Autodesk Inventor part; units mm, degrees
ref_plane "YZ Plane" through (0, 0, 0) normal (1, 0, 0) x (0, 1, 0)
ref_plane "XZ Plane" through (0, 0, 0) normal (0, 1, 0) x (-1, 0, 0)
ref_plane "XY Plane" through (0, 0, 0) normal (0, 0, 1) x (1, 0, 0)
sketch "本体面" plane through (0, 0, 0) normal (0, 0, 1) x (1, 0, 0)
  line L0 (-13.7, 10) -> (13.7, 10)
  line L1 (13.7, 10) -> (13.7, 0)
  line L2 (13.7, 0) -> (-13.7, 0)
  line L3 (-13.7, 0) -> (-13.7, 10)
  point P0 (0, 0)
  point P1 (0, 0)
  dimension "d0" = 27.4
  dimension "d1" = 10
extrude "本体" add sketch "本体面" along normal blind 42
sketch "空洞面" plane through (0, 0, 42) normal (0, 0, 1) x (1, 0, 0)
  line L0 (-11.9, 10) -> (11.9, 10)
  line L1 (11.9, 10) -> (11.9, 3.5)
  line L2 (9.9, 1.5) -> (-9.9, 1.5)
  line L3 (-11.9, 3.5) -> (-11.9, 10)
  line L4 (13.7, 10) -> (-13.7, 10)
  arc A0 (-11.9, 3.5) -> (-9.9, 1.5) centre (-9.9, 3.5) ccw
  arc A1 (9.9, 1.5) -> (11.9, 3.5) centre (9.9, 3.5) ccw
  point P0 (0, 0)
  point P1 (11.9, 1.5)
  point P2 (-11.9, 1.5)
  point P3 (0, 10)
  dimension "d4" = 23.8
  dimension "d5" = 8.5
  dimension "d6" = 2
extrude "空洞" cut sketch "空洞面" against normal blind 42
sketch "左溝面" plane through (0, 0, 42) normal (0, 0, 1) x (1, 0, 0)
  line L0 (-12.9, 9.2) -> (-11.9, 9.2)
  line L1 (-11.9, 9.2) -> (-11.9, 7.2)
  line L2 (-11.9, 7.2) -> (-12.9, 7.2)
  line L3 (-12.9, 7.2) -> (-12.9, 9.2)
  line L4 (-11.9, 10) -> (-13.7, 10) construction
  line L5 (-13.7, 10) -> (-13.7, 0) construction
  line L6 (-11.9, 3.5) -> (-11.9, 10) construction
  point P0 (0, 0)
  dimension "d10" = 2
  dimension "d27" = 0.8
  dimension "d28" = 0.8
extrude "左溝" cut sketch "左溝面" against normal blind 41
sketch "右溝面" plane through (0, 0, 42) normal (0, 0, 1) x (1, 0, 0)
  line L0 (11.9, 9.2) -> (12.9, 9.2)
  line L1 (12.9, 9.2) -> (12.9, 7.2)
  line L2 (12.9, 7.2) -> (11.9, 7.2)
  line L3 (11.9, 7.2) -> (11.9, 9.2)
  line L4 (13.7, 10) -> (11.9, 10)
  line L5 (13.7, 0) -> (13.7, 10)
  line L6 (11.9, 10) -> (11.9, 3.5)
  point P0 (0, 0)
  dimension "d22" = 2
  dimension "d29" = 0.8
  dimension "d30" = 0.8
extrude "右溝" cut sketch "右溝面" against normal blind 41
sketch "右穴位置" plane through (13.7, 0, 0) normal (1, 0, 0) x (0, 0, -1)
  line L0 (-20, 0) -> (0, 0) construction
  line L1 (-20, 0) -> (-20, 4) construction
  line L2 (0, 10) -> (-42, 10) construction
  line L3 (0, 0) -> (-42, 0) construction
  line L4 (0, 10) -> (0, 0) construction
  dimension "d31" = 20
  dimension "d32" = 4
hole "右穴" at (13.7, 4, 20) direction (-1, 0, 0) diameter 2.5 depth 8 tip angle 118
sketch "左穴位置" plane through (-13.7, 0, 0) normal (-1, 0, 0) x (0, 0, 1)
  line L0 (0, 0) -> (20, 0) construction
  line L1 (20, 0) -> (20, 4) construction
  point P0 (0, 0)
  point P1 (0, 0)
  dimension "d40" = 4
  dimension "d41" = 20
hole "左穴" at (-13.7, 4, 20) direction (1, 0, 0) diameter 2.5 depth 8 tip angle 118
sketch "背穴位置" plane through (-13.7, 0, 0) normal (0, -1, 0) x (1, 0, 0)
  line L0 (13.7, 20) -> (13.7, 0) construction
  line L1 (27.4, 0) -> (0, 0) construction
  dimension "d49" = 20
hole "背穴" at (0, 0, 20) direction (0, 1, 0) diameter 2.5 depth 8 tip angle 118
properties part number "Pcam5C_holder"
The listing builds one solid part. Answer for the finished solid, in the listing's coordinates (mm). A direction names the side the tool comes from. Round coordinates to 2 decimals unless told otherwise and drop trailing zeros. Write each loop counter-clockwise with the first axis right and the second up, starting at its lowest first coordinate (ties: lowest second). Pieces come first, ordered by that corner, then holes. Notation, with made-up numbers: (88.5, 17) - (93.5, 17) arc R31 ccw to (93.5, 41) - close; hole circle Ø7 at (81, 18). An arc over 180 degrees is marked (long way). Use a Markdown table: item, result. Add a question column.
1. A tool of negligible diameter and unlimited length cuts with its end or side. For faces 4 (the face through (-12.4, 8.2, 1)), 5 (the face through (11.3, 2.07, 21.29)), 6 (the face through (0.479, 0.76, 18.845)), from which of +Z, -Z, +X, -X, +Y, -Y can it reach the whole face along a straight path? Write none if from no direction.
2. A flat-ended cylindrical pin translates along its axis: P1, Ø2, axis at x = -5, z = 31, coming from the +Y side. Find the tip coordinate at first contact, or state that the pin passes through.
3. For a pull along X with two mould halves and no side action, classify faces 1 (the face through (12.713, 2.946, 19.328)), 2 (the face through (13.7, 5, 21)), 3 (the face through (12.9, 8, 22)) as +X half, -X half, draft (parallel to the pull), parting line (faces both ways), or undercut.
4. The part is cut by section A-A (z = 20). Write down the section's boundary in (x, y), and give its area (3 significant figures).
5. Consider line 1 (Y direction, x = 12.7, z = 20); line 2 (Z direction, x = -12.95, y = 4); line 3 (X direction, y = 0.5, z = 20). Determine where each line is inside the solid, lowest interval first.
6. The part is cut by section B-B (x = 0). Write down the section's boundary in (y, z), and give its area (4 significant figures).
7. The part is cut by section C-C (y = 4.75). Write down the section's boundary in (x, z), and give its area (3 significant figures).
Reported:
| question | item | result |
|---|---|---|
| 1 | face 4 | +Z |
| 1 | face 5 | +Z, -Z, +Y |
| 1 | face 6 | +Y, -Y |
| 2 | P1 | y = 1.5 |
| 3 | face 1 | draft |
| 3 | face 2 | +X half |
| 3 | face 3 | undercut |
| 4 | outline | (-13.7, 0) - (-1.25, 0) - (-1.25, 1.5) - (-9.9, 1.5) arc R2 cw to (-11.75, 2.75) - (-13.7, 2.75) - close; (-13.7, 5.25) - (-11.9, 5.25) - (-11.9, 7.2) - (-12.9, 7.2) - (-12.9, 9.2) - (-11.9, 9.2) - (-11.9, 10) - (-13.7, 10) - close; (1.25, 0) - (13.7, 0) - (13.7, 2.75) - (11.75, 2.75) arc R2 cw to (9.9, 1.5) - (1.25, 1.5) - close; (11.9, 5.25) - (13.7, 5.25) - (13.7, 10) - (11.9, 10) - (11.9, 9.2) - (12.9, 9.2) - (12.9, 7.2) - (11.9, 7.2) - close |
| 4 | area | 56.6 mm^2 |
| 5 | line 1 | 0 to 2.75, 5.25 to 7.2, 9.2 to 10 |
| 5 | line 2 | 0 to 18.75, 21.25 to 42 |
| 5 | line 3 | -13.7 to -1.25, 1.25 to 13.7 |
| 6 | outline | (0, 0) - (1.5, 0) - (1.5, 18.75) - (0, 18.75) - close; (0, 21.25) - (1.5, 21.25) - (1.5, 42) - (0, 42) - close |
| 6 | area | 59.25 mm^2 |
| 7 | outline | (-13.7, 0) - (-11.9, 0) - (-11.9, 19) - (-13.7, 19) - close; (-13.7, 21) - (-11.9, 21) - (-11.9, 42) - (-13.7, 42) - close; (11.9, 0) - (13.7, 0) - (13.7, 19) - (11.9, 19) - close; (11.9, 21) - (13.7, 21) - (13.7, 42) - (11.9, 42) - close |
| 7 | area | 144 mm^2 |
